The model under review builds one solid part; all positions refer to its coordinate system, in mm. Face numbers are marked on the shaded views. A direction names the side the tool comes from. Coordinates: 2 decimals unless noted, no trailing zeros. Loops run counter-clockwise (first coordinate to the right, second up) from the corner with the lowest first, then second, coordinate; pieces in that order, holes last. Notation, with made-up numbers: M -22,-31.5 L -11,-31.5 A22 ccw -11,-4.5 Z; hole C -35.75,22 d7. An arc over 180 degrees is marked long. Return JSON: item names as keys, results as strings.
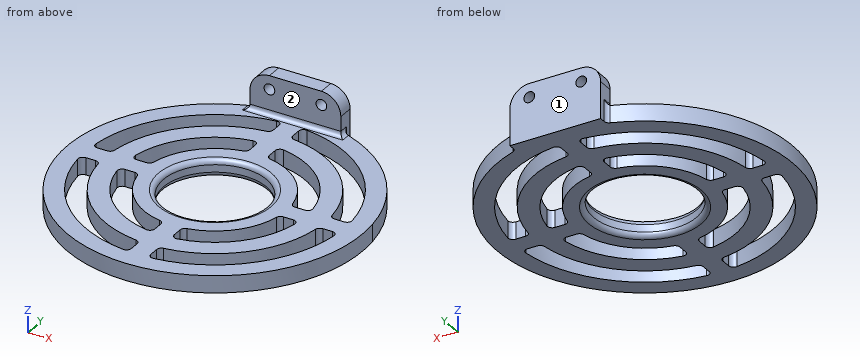
Autodesk Inventor part; units mm, degrees
ref_plane "Work Plane1" through (0, 0, 5.588) normal (0, 0, 1) x (1, 0, 0)
ref_plane "Work Plane2" through (-8.5, -5.08, 18.288) normal (0, -1, 0) x (1, 0, 0)
ref_plane "YZ Plane" through (0, 0, 0) normal (1, 0, 0) x (0, 1, 0)
sketch "Sketch1" plane through (0, 0, 0) normal (0, 0, 1) x (1, 0, 0)
  line L0 (3, 0) -> (-3, 0)
  line L1 (0, 0) -> (13.85, 0)
  line L2 (14.85, -3.0647) -> (14.85, -1)
  line L3 (14.85, -3.0647) -> (14.85, -1)
  line L4 (0, 0) -> (-13.85, 0)
  line L5 (13.85, 0) -> (-13.85, 0)
  line L6 (-14.85, -3.0647) -> (-14.85, -1)
  line L7 (-14.85, -3.0647) -> (-14.85, -1)
  arc A0 (47.8846, -42.8653) -> (14.85, -3.0647) centre (0, -49) ccw
  arc A1 (-14.85, -3.0647) -> (14.85, -3.0647) centre (0, -49) ccw
  line L8 (-14.85, -1) -> (-14.85, 0)
  line L9 (-14.85, 0) -> (-13.85, 0)
  line L10 (14.85, -1) -> (14.85, 0)
  line L11 (14.85, 0) -> (13.85, 0)
  circle A2 centre (0, -49) radius 16.8275
  line L12 (-3.175, -26.041) -> (-3.175, -19.6437)
  line L13 (-3.175, -13.2633) -> (-3.175, -6.892)
  line L14 (3.175, -26.041) -> (3.175, -19.6437)
  line L15 (3.175, -13.2633) -> (3.175, -6.892)
  arc A3 (-3.175, -26.041) -> (-22.959, -45.825) centre (0, -49) ccw
  arc A4 (-3.175, -19.6437) -> (-29.3563, -45.825) centre (0, -49) ccw
  line L16 (-22.959, -45.825) -> (-29.3563, -45.825)
  line L17 (-35.7367, -45.825) -> (-42.108, -45.825)
  line L18 (-22.959, -52.175) -> (-29.3563, -52.175)
  line L19 (-35.7367, -52.175) -> (-42.108, -52.175)
  arc A5 (-3.175, -13.2633) -> (-35.7367, -45.825) centre (0, -49) ccw
  arc A6 (-3.175, -6.892) -> (-42.108, -45.825) centre (0, -49) ccw
  arc A7 (-22.959, -52.175) -> (-3.175, -71.959) centre (0, -49) ccw
  arc A8 (-29.3563, -52.175) -> (-3.175, -78.3563) centre (0, -49) ccw
  line L20 (-3.175, -71.959) -> (-3.175, -78.3563)
  line L21 (-3.175, -84.7367) -> (-3.175, -91.108)
  line L22 (3.175, -71.959) -> (3.175, -78.3563)
  line L23 (3.175, -84.7367) -> (3.175, -91.108)
  arc A9 (-35.7367, -52.175) -> (-3.175, -84.7367) centre (0, -49) ccw
  arc A10 (-42.108, -52.175) -> (-3.175, -91.108) centre (0, -49) ccw
  arc A11 (3.175, -71.959) -> (22.959, -52.175) centre (0, -49) ccw
  arc A12 (22.959, -45.825) -> (3.175, -26.041) centre (0, -49) ccw
  arc A13 (3.175, -78.3563) -> (29.3563, -52.175) centre (0, -49) ccw
  arc A14 (29.3563, -45.825) -> (3.175, -19.6437) centre (0, -49) ccw
  line L24 (22.959, -45.825) -> (29.3563, -45.825)
  line L25 (35.7367, -45.825) -> (42.108, -45.825)
  line L26 (22.959, -52.175) -> (29.3563, -52.175)
  line L27 (35.7367, -52.175) -> (42.108, -52.175)
  arc A15 (3.175, -84.7367) -> (35.7367, -52.175) centre (0, -49) ccw
  arc A16 (35.7367, -45.825) -> (3.175, -13.2633) centre (0, -49) ccw
  arc A17 (3.175, -91.108) -> (42.108, -52.175) centre (0, -49) ccw
  arc A18 (42.108, -45.825) -> (3.175, -6.892) centre (0, -49) ccw
  point P0 (0, 0)
  point P1 (-16.85, -4.0995)
ref_plane "Work Plane1" through (0, 0, 5.588) normal (0, 0, 1) x (1, 0, 0)
sketch "Sketch3" plane through (0, 0, 5.588) normal (0, 0, 1) x (1, 0, 0)
  line L0 (14.85, 0) -> (-14.85, 0)
  line L1 (-14.85, 0) -> (14.85, 0)
  line L2 (14.85, 0) -> (14.85, -5.08)
  line L3 (14.85, -5.08) -> (-14.85, -5.08)
  line L4 (-14.85, -5.08) -> (-14.85, 0)
  point P0 (0, 0)
  dimension "d16" = 5.08
extrude "Extrusion2" add sketch "Sketch3" along normal blind 12.7
ref_plane "Work Plane2" through (-8.5, -5.08, 18.288) normal (0, -1, 0) x (1, 0, 0)
sketch "Sketch4" plane through (-8.5, -5.08, 18.288) normal (0, -1, 0) x (1, 0, 0)
  line L0 (17, 0) -> (0, 0)
  circle A0 centre (0, -4.445) radius 1.75
  circle A1 centre (17, -4.445) radius 1.75
  point P0 (8.5, -18.288)
  dimension "d22" = 3.5
  dimension "d23" = 3.5
extrude "Extrusion3" cut sketch "Sketch4" against normal blind 10.16
extrude "Extrusion4" add sketch "Sketch1" along normal blind 5.588
fillet "Fillet5" radius 6.35 2 edges at (-14.85, -2.54, 18.288) (14.85, -2.54, 18.288)
fillet "Fillet6" radius 1.5875 5 edges at (0, -5.08, 5.588) (14.85, -3.0647, 2.794) (14.85, -4.0724, 5.588) (-14.85, -3.0647, 2.794) (-14.85, -4.0724, 5.588)
fillet "Fillet7" radius 1.5875 34 edges at (-3.175, -6.892, 2.794) (-3.175, -13.2633, 2.794) (-3.175, -19.6437, 2.794) (-3.175, -26.041, 2.794) (-42.108, -45.825, 2.794) (-35.7367, -45.825, 2.794) (-29.3563, -45.825, 2.794) (-22.959, -45.825, 2.794) (-42.108, -52.175, 2.794) (-35.7367, -52.175, 2.794) (-29.3563, -52.175, 2.794) (-22.959, -52.175, 2.794) (-3.175, -71.959, 2.794) (-3.175, -78.3563, 2.794) (-3.175, -84.7367, 2.794) (-3.175, -91.108, 2.794) (3.175, -91.108, 2.794) (3.175, -84.7367, 2.794) (3.175, -78.3563, 2.794) (3.175, -71.959, 2.794) (22.959, -52.175, 2.794) (29.3563, -52.175, 2.794) (35.7367, -52.175, 2.794) (42.108, -52.175, 2.794) (42.108, -45.825, 2.794) (35.7367, -45.825, 2.794) (29.3563, -45.825, 2.794) (22.959, -45.825, 2.794) (3.175, -26.041, 2.794) (3.175, -19.6437, 2.794) (3.175, -13.2633, 2.794) (3.175, -6.892, 2.794) (-16.8275, -49, 0) (-16.8275, -49, 5.588)
properties part number "backSideThrusterCover"
1. Machinability: for the marked faces 1 and 2, which of the approach directions +Z, -Z, +X, -X, +Y, -Y give a long, thin tool a straight path to every point of the face, cutting with its end or side? Answer none if there is none.
Check values:
{"face 1": "+Z, -Z, +X, -X, +Y", "face 2": "+Z, +X, -X, -Y"}
2. Add section B-B on y = -49. Give the boundary of the cut face in (x, z) (1 decimal).
Check values:
{"outline": "M -48.3,0 L -18.4,0 A1.6 ccw -16.8,1.6 L -16.8,4 A1.6 ccw -18.4,5.6 L -48.3,5.6 Z; M 16.8,1.6 A1.6 ccw 18.4,0 L 48.3,0 L 48.3,5.6 L 18.4,5.6 A1.6 ccw 16.8,4 Z"}
3. To check wall thickness, follow line 1 (Y direction, x = 0, z = 2.5); line 2 (Y direction, x = 18, z = 3.5); line 3 (Y direction, x = -4, z = 2.5). State the ranges of each line that lie inside material, in increasing order.
Check values:
{"line 1": "-97.28 to -65.83, -32.17 to 0", "line 2": "-93.79 to -87.2, -80.04 to -72.41, -63.6 to -34.4, -25.59 to -17.96, -10.8 to -4.21", "line 3": "-97.11 to -90.75, -84.77 to -77.92, -71.91 to -65.35, -32.65 to -26.09, -20.08 to -13.23, -7.25 to 0"}
4. Insertion check: pin 1 Ø1.6 at (y, z) = (-10, 2.5) entering from -X; pin 2 Ø1.5 at (x, z) = (-6.5, 15.5) entering from -Y; pin 3 Ø4 at (x, z) = (20.5, 2) entering from +Y; pin 4 Ø5 at (x, y) = (30, -75.5) entering from -Z. Each pin has a flat end and moves straight along its axis. Give the tip position at first contact, or say it passes through.
Check values:
{"pin 1": "x = -29.52", "pin 2": "y = -5.08", "pin 3": "y = -4.41", "pin 4": "z = 0"}
5. Add section A-A on x = 0. Give the boundary of the cut face in (y, z) (1 decimal), plus the area to 3 significant figures.
Check values:
{"outline": "M -97.3,0 L -67.4,0 A1.6 ccw -65.8,1.6 L -65.8,4 A1.6 ccw -67.4,5.6 L -97.3,5.6 Z; M -32.2,1.6 A1.6 ccw -30.6,0 L 0,0 L 0,18.3 L -5.1,18.3 L -5.1,7.2 A1.6 cw -6.7,5.6 L -30.6,5.6 A1.6 ccw -32.2,4 Z", "area": "418 mm²"}
6. Add section C-C on x = -20.5. Give the boundary of the cut face in (y, z), plus the area to 3 significant figures.
Check values:
{"outline": "M -92.71,0 L -85.92,0 L -85.92,5.59 L -92.71,5.59 Z; M -78.44,0 L -70.25,0 L -70.25,5.59 L -78.44,5.59 Z; M -59.81,0 L -38.19,0 L -38.19,5.59 L -59.81,5.59 Z; M -27.75,0 L -19.56,0 L -19.56,5.59 L -27.75,5.59 Z; M -12.08,0 L -5.29,0 L -5.29,5.59 L -12.08,5.59 Z", "area": "288 mm²"}
7. Add section D-D on y = -59.5. State how many separate pieces and enclosed holes the cut face has, plus the area to 3 significant figures.
Check values:
{"separate pieces": "6", "enclosed holes": "0", "area": "226 mm²"}
